```python
from build123d import *

# Parameters (mm, degrees)
SKETCH_1_R          = 42
EXTRUDE_1_DEPTH     = 5
SKETCH_2_W          = 11
SKETCH_2_H          = 11
EXTRUDE_2_DEPTH     = 5
SKETCH_4_R          = 6
CUT_EXTRUDE_1_DEPTH = 25
SKETCH_5_R          = 9
CUT_EXTRUDE_2_DEPTH = 9
CUT_EXTRUDE_START   = 8
SKETCH_6_R          = 10
SKETCH_6_R_2        = 9
CUT_EXTRUDE_3_DEPTH = 1.5
SKETCH_7_R          = 30
CUT_EXTRUDE_4_DEPTH = 30
FILLET_1_R          = 2


with BuildPart() as part:
    # Sketch 1 → Extrude 1 (new body)
    with BuildSketch(Plane.XY):
        Circle(SKETCH_1_R)
    extrude(amount=EXTRUDE_1_DEPTH)



with BuildPart() as body_2:
    # Sketch 2 → Revolve 1 (revolve)
    with BuildSketch(Plane.XY.offset(5), mode=Mode.PRIVATE) as revolve_1_sk:
        with Locations((94.5, -0.125)):
            Rectangle(SKETCH_2_W, SKETCH_2_H)
    revolve(revolve_1_sk.sketch.rotate(Axis((100, 22.717290725, 5), (0, -1, 0)), 270), axis=Axis((100, 22.717290725, 5), (0, -1, 0)))


with BuildPart() as part_1:
    add(part.part)

    add(body_2.part)  # Extrude 2 merges body 2
    # Sketch 3 → Extrude 2 (add, symmetric)
    with BuildSketch(Plane.XY.offset(5)):
        with BuildLine():
            Line((17.314737244, 38.264864748), (90, 5.375))
            Line((90, 5.375), (90, -4))
            Line((90, -4), (17.911593748, -37.989140678))
            ThreePointArc((17.911593748, -37.989140678), (-41.998713488, -0.328732965), (17.314737244, 38.264864748))
        make_face()
    extrude(amount=EXTRUDE_2_DEPTH, both=True)

    # Sketch 4 → Cut-Extrude 1 (cut)
    with BuildSketch(Plane.XZ.offset(5.625)):
        with Locations(Location((100, 5, 0), (0, 0, 270))):
            Circle(SKETCH_4_R)
    extrude(amount=-CUT_EXTRUDE_1_DEPTH, mode=Mode.SUBTRACT)

    # Sketch 5 → Cut-Extrude 2 (cut)
    with BuildSketch(Plane.XZ.offset(5.625)):
        with Locations(Location((100, 5, 0), (0, 0, 270))):
            Circle(SKETCH_5_R)
    extrude(amount=-CUT_EXTRUDE_2_DEPTH, mode=Mode.SUBTRACT)

    # Sketch 6 → Cut-Extrude 3 (cut)
    # profile 1 of 2: a face of its own
    with BuildSketch(Plane.XZ.offset(-3.375).offset(CUT_EXTRUDE_START)):
        with Locations(Location((100, 5, 0), (0, 0, 270))):
            Circle(SKETCH_6_R)
        with Locations(Location((100, 5, 0), (0, 0, 270))):
            Circle(SKETCH_6_R_2, mode=Mode.SUBTRACT)
    # profile 2 of 2: a face of its own
    with BuildSketch(Plane.XZ.offset(-3.375).offset(CUT_EXTRUDE_START)):
        with Locations(Location((100, 5, 0), (0, 0, 270))):
            Circle(SKETCH_6_R_2)
    extrude(amount=-CUT_EXTRUDE_3_DEPTH, mode=Mode.SUBTRACT)

    # Sketch 7 → Cut-Extrude 4 (cut)
    with BuildSketch(Plane.XY.offset(10)):
        Circle(SKETCH_7_R)
        with BuildLine():
            Line((26.356552806, -27.373931471), (75.930900201, -4))
            Line((75.930900201, -4), (37.788887255, -4))
            ThreePointArc((37.788887255, -4), (34.135678377, -16.695971422), (26.356552806, -27.373931471))
        make_face()
        with BuildLine():
            Line((37.788887255, 4), (75.930900201, 4))
            Line((75.930900201, 4), (26.356552806, 27.373931471))
            ThreePointArc((26.356552806, 27.373931471), (34.135678377, 16.695971422), (37.788887255, 4))
        make_face()
    extrude(amount=-CUT_EXTRUDE_4_DEPTH, mode=Mode.SUBTRACT)

    # Fillet 1
    fillet_1_edges = [part_1.edges().sort_by_distance(p)[0] for p in [
        (37.788887255, 4, 5),
        (26.356552806, 27.373931471, 5),
        (75.930900201, 4, 5),
        (26.356552806, -27.373931471, 5),
        (37.788887255, -4, 5),
        (75.930900201, -4, 5),
    ]]
    fillet(fillet_1_edges, radius=FILLET_1_R)


solid = part_1.part
```
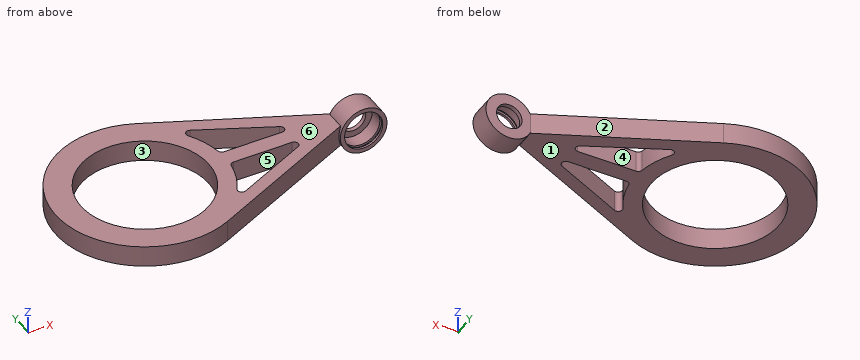
Work out the finished part from the listing and answer in its coordinate system (mm). Face numbers are marked on the shaded views. A direction names the side the tool comes from. Give positions to 0.01 mm unless a question says otherwise; leave off trailing zeros. Order: outer loops, then holes, each group sorted by start corner. A loop starts at its lowest first (then second) coordinate and runs counter-clockwise, first axis right, second up. Notation, with made-up numbers: M 60,32.25 L 67,32.25 A6 cw 67,43.25 Z; hole C 73,-13.5 d5. An arc over 180 degrees is marked long. Return JSON: item names as keys, results as strings.
1) Each of these flat-tipped pins is pushed along its axis until it touches: pin 1 (1 mm diameter, centred on x = 35.5, y = -29.5, fed in from -Z); pin 2 (5 mm diameter, centred on y = 20, z = 10.5, fed in from +X); pin 3 (6 mm diameter, centred on x = 99, z = 1, fed in from -Y) (3 decimals); pin 4 (1.5 mm diameter, centred on x = 21, z = -2, fed in from +Y) (1 decimal). Where does it stop, or does it pass through?
Resolved:
{"pin 1": "z = 0", "pin 2": "x = 63.09", "pin 3": "y = 3.375", "pin 4": "through"}
2) Section A-A, the plane y = 0 is taken. Write down the section's boundary in (x, z), plus the area to 3 significant figures.
Resolved:
{"outline": "M -42,0 L -30,0 L -30,10 L -42,10 Z; M 30,0 L 90,0 L 90,0.42 A11 ccw long 90,9.58 L 90,10 L 30,10 Z; hole C 100,5 d18", "area": "839 mm^2"}
3) Straight lines are drawn through the part: line 1 along X through (y, z) = (-0.75, 5); line 2 along X through (y, z) = (5, 5); line 3 along X through (y, z) = (4.7, 5). For each, find the intervals that lie inside material, in ascending order. Write a range as [from, to].
Resolved:
{"line 1": "[-41.99, -29.99], [29.99, 91], [109, 111]", "line 2": "[-41.7, -29.58], [29.58, 37.82], [68.73, 94], [106, 111]", "line 3": "[-41.74, -29.63], [29.63, 38.03], [68.52, 94], [106, 111]"}
4) Section B-B, the plane x = 0 is taken. Write down the section's boundary in (y, z).
Resolved:
{"outline": "M -42,0 L -30,0 L -30,10 L -42,10 Z; M 30,0 L 42,0 L 42,10 L 30,10 Z"}
5) For a pull along X with two mould halves and no side action, classify the marked faces 1, 2, 3 and 4 as +X half, -X half, draft (parallel to the pull), parting line (faces both ways), or undercut.
Resolved:
{"face 1": "draft", "face 2": "+X half", "face 3": "undercut", "face 4": "undercut"}
6) Section D-D, the plane x = 100 is taken. Write down the section's boundary in (y, z) (3 decimals).
Resolved:
{"outline": "M -5.625,-6 L 5.375,-6 L 5.375,-1 L 3.375,-1 L 3.375,-4 L -3.125,-4 L -3.125,-5 L -4.625,-5 L -4.625,-4 L -5.625,-4 Z; M -5.625,14 L -4.625,14 L -4.625,15 L -3.125,15 L -3.125,14 L 3.375,14 L 3.375,11 L 5.375,11 L 5.375,16 L -5.625,16 Z"}
7) A tool of negligible diameter and unlimited length cuts with its end or side. For the marked faces 5 and 6, from which of +Z, -Z, +X, -X, +Y, -Y can it reach the whole face along a straight path? Write none if from no direction.
Resolved:
{"face 5": "+Z, -Z", "face 6": "+Z, -X, +Y, -Y"}
8) Section C-C, the plane z = 8 is taken. Give the number of separate pieces and of enclosed holes in the cut face, plus the area to 3 significant figures.
Resolved:
{"separate pieces": "2", "enclosed holes": "3", "area": "3,770 mm^2"}
